CAD build for the part. Positions are in the model's coordinates, mm. A direction names the side the tool comes from. Give positions to 0.01 mm unless a question says otherwise; leave off trailing zeros. Write each loop counter-clockwise with the first axis right and the second up, starting at its lowest first coordinate (ties: lowest second). Pieces come first, ordered by that corner, then holes. Notation, with made-up numbers: (25.25, 5) -> (73.25, 5) arc R23 ccw to (73.25, 27) -> close; hole circle Ø3 at (-24, -16). An arc over 180 degrees is marked (long way). Answer in a Markdown table with one row per item. Add a question column.
```python
from build123d import *

# Parameters (mm, degrees)
SKETCH_1_R      = 1.95
SKETCH_1_R_2    = 1.45
SKETCH_1_W      = 40
SKETCH_1_H      = 80
EXTRUDE_1_DEPTH = 3
FILLET_1_R      = 5
FILLET_3_R      = 2


with BuildPart() as part:
    # 草图1 → 凸台-拉伸1 (new body)
    with BuildSketch(Plane(origin=(0, 0, 0), x_dir=(1, 0, 0), z_dir=(0, 1, 0))):
        Polygon((-60, -50), (-60, 50), (60, 50), (60, -19.7), (80, -29.7), (80, -44.7), (60, -54.7), (45, -54.7), (45, -50), align=None)
        with Locations(Location((-33.6, 21, 0), (0, 0, 270))):
            Circle(SKETCH_1_R, mode=Mode.SUBTRACT)
        with Locations(Location((-33.6, -21, 0), (0, 0, 90))):
            Circle(SKETCH_1_R, mode=Mode.SUBTRACT)
        with Locations(Location((33.6, -21, 0), (0, 0, 270))):
            Circle(SKETCH_1_R, mode=Mode.SUBTRACT)
        with Locations(Location((33.6, 21, 0), (0, 0, 90))):
            Circle(SKETCH_1_R, mode=Mode.SUBTRACT)
        with Locations(Location((65, -37.2, 0), (0, 0, 270))):
            Circle(SKETCH_1_R_2, mode=Mode.SUBTRACT)
        with Locations(Location((75, -37.2, 0), (0, 0, 270))):
            Circle(SKETCH_1_R_2, mode=Mode.SUBTRACT)
        with Locations(Location((52.5, -24.7, 0), (0, 0, 270))):
            Circle(SKETCH_1_R_2, mode=Mode.SUBTRACT)
        with Locations(Location((52.5, -49.7, 0), (0, 0, 270))):
            Circle(SKETCH_1_R_2, mode=Mode.SUBTRACT)
        with Locations(Location((52.5, 0, 0), (0, 0, 270))):
            Circle(SKETCH_1_R_2, mode=Mode.SUBTRACT)
        with Locations(Location((-52.5, 0, 0), (0, 0, 90))):
            Circle(SKETCH_1_R_2, mode=Mode.SUBTRACT)
        with Locations(Location((-52.5, -24.7, 0), (0, 0, 90))):
            Circle(SKETCH_1_R_2, mode=Mode.SUBTRACT)
        with Locations(Location((-52.5, 24.7, 0), (0, 0, 270))):
            Circle(SKETCH_1_R_2, mode=Mode.SUBTRACT)
        with Locations(Location((52.5, 24.7, 0), (0, 0, 90))):
            Circle(SKETCH_1_R_2, mode=Mode.SUBTRACT)
        Rectangle(SKETCH_1_W, SKETCH_1_H, mode=Mode.SUBTRACT)
    extrude(amount=EXTRUDE_1_DEPTH)

    # 圆角1
    fillet_1_edges = [part.edges().sort_by_distance(p)[0] for p in [
        (60, 1.5, 19.7),
        (80, 1.5, 29.7),
        (80, 1.5, 44.7),
        (60, 1.5, 54.7),
        (-60, 1.5, 50),
        (-60, 1.5, -50),
        (60, 1.5, -50),
        (20, 1.5, 40),
        (20, 1.5, -40),
        (-20, 1.5, -40),
        (-20, 1.5, 40),
    ]]
    fillet(fillet_1_edges, radius=FILLET_1_R)

    # 圆角3
    fillet_3_edges = [part.edges().sort_by_distance(p)[0] for p in [
        (45, 1.5, 54.7),
        (45, 1.5, 50),
    ]]
    fillet(fillet_3_edges, radius=FILLET_3_R)


solid = part.part
```
Item 1: Slice it at D-D, the plane z = -6.5. List the corners of the cut face in (x, y).
Item 2: Slice it at C-C, the plane x = -52.5. List the corners of the cut face in (y, z).
Item 3: Probe L1, parallel to X at y = 2.3, z = -21; L2, parallel to X at y = 1.85, z = 0; L3, parallel to X at y = 0.95, z = -12.5. List the from-to ranges inside material, lowest first. Write a range as from..to.
Item 4: Drop flat-ended pins along their axis: pin 1 Ø0.9 at (y, z) = (2, -25) entering from +X; pin 2 Ø1.5 at (x, y) = (-11.5, 1.5) entering from +Z; pin 3 Ø2.5 at (x, z) = (52.5, -24.7) entering from +Y. Give the stop position or say it passes through.
Item 5: Mould opens along Z. For faces 4 (the face through (19, 2, 38)), 5 (the face through (-5, 1, 50)), 6 (the face through (80, 1, 37)) say: released by +Z, released by -Z, zero draft, split by the parting line, or undercut.
Item 6: Slice it at A-A, the plane x = -3. List the corners of the cut face in (y, z), then the cut area to 3 significant figures.
Item 7: Slice it at B-B, the plane z = -21. List the corners of the cut face in (x, y).
Item 8: Which spindle directions (+Z, -Z, +X, -X, +Y, -Y) get a long thin tool onto all of the face, cutting with end or side? Do faces 1 (the face through (60, 1, -15)), 2 (the face through (-19, 2, -38)), 3 (the face through (27, 3, 2)). Say none if no direction does.
Answer key:
| question | item | result |
|---|---|---|
| 1 | outline | (-60, 0) -> (-20, 0) -> (-20, 3) -> (-60, 3) -> close; (20, 0) -> (60, 0) -> (60, 3) -> (20, 3) -> close |
| 2 | outline | (0, -50) -> (3, -50) -> (3, -26.15) -> (0, -26.15) -> close; (0, -23.25) -> (3, -23.25) -> (3, -1.45) -> (0, -1.45) -> close; (0, 1.45) -> (3, 1.45) -> (3, 23.25) -> (0, 23.25) -> close; (0, 26.15) -> (3, 26.15) -> (3, 50) -> (0, 50) -> close |
| 3 | L1 | x = -60..-35.55, -31.65..-20, 20..31.65, 35.55..60 |
| 3 | L2 | x = -60..-53.95, -51.05..-20, 20..51.05, 53.95..60 |
| 3 | L3 | x = -60..-20, 20..60 |
| 4 | pin 1 | stops at x = 60 |
| 4 | pin 2 | stops at z = 50 |
| 4 | pin 3 | passes through |
| 5 | face 4 | undercut |
| 5 | face 5 | released by +Z |
| 5 | face 6 | zero draft |
| 6 | outline | (0, -50) -> (3, -50) -> (3, -40) -> (0, -40) -> close; (0, 40) -> (3, 40) -> (3, 50) -> (0, 50) -> close |
| 6 | area | 60.0 mm² |
| 7 | outline | (-60, 0) -> (-35.55, 0) -> (-35.55, 3) -> (-60, 3) -> close; (-31.65, 0) -> (-20, 0) -> (-20, 3) -> (-31.65, 3) -> close; (20, 0) -> (31.65, 0) -> (31.65, 3) -> (20, 3) -> close; (35.55, 0) -> (60, 0) -> (60, 3) -> (35.55, 3) -> close |
| 8 | face 1 | -Z, +X, +Y, -Y |
| 8 | face 2 | +Y, -Y |
| 8 | face 3 | +Z, -Z, +X, -X, +Y |
